Read the model definition and answer for the solid it produces. Units are mm, in the model's axes. A direction names the side the tool comes from. Coordinates: 2 decimals unless noted, no trailing zeros. Order: outer loops, then holes, each group sorted by start corner. A loop starts at its lowest first (then second) coordinate and runs counter-clockwise, first axis right, second up. Notation, with made-up numbers: (7.25, 0) -> (42.25, 0) arc R27 cw to (42.25, 23) -> close; hole circle Ø3 at (6.25, 19.25). An arc over 180 degrees is marked (long way). Answer as a JSON object with one key per item and string values. Group by question number.
1) Section D-D on x = 1 is taken. Determine the outline of the cut face in (y, z) (3 decimals), and give its area (3 significant figures).
2) A tool of negligible diameter and unlimited length cuts with its end or side. For faces 1 (the flat face through (1.5, 2.4, 9.2)), 2 (the flat face through (3, 2.875, 10)), 3 (the flat face through (5, 2.4, 9.2)), 4 (the flat face through (3, -2.375, 10)), from which of +Z, -Z, +X, -X, +Y, -Y can it reach the whole face along a straight path? Write none if from no direction.
3) Section A-A on z = -3.95 is taken. Determine the outline of the cut face in (x, y) (3 decimals).
4) Consider L1, parallel to Z at x = 5.25, y = 0; L2, parallel to Y at x = 2, z = -3.95 (3 decimals); L3, parallel to Y at x = 4.5, z = 6.75 (3 decimals). Determine where each line is inside the solid, lowest interval first.
5) Section B-B on x = 2.75 is taken. Determine the outline of the cut face in (y, z) (3 decimals), and give its area (3 significant figures).
6) Section C-C on y = 0 is taken. Determine the outline of the cut face in (x, z).
7) Determine the mould class of faces 5 (the flat face through (3, 1.875, 10)), 6 (the cylindrical face through (4.715, 2.368, 12.649)), 7 (the flat face through (3, 0, -6.45)), 8 (the cylindrical face through (3.204, -0.217, -2.974)) for opening direction Z: released by +Z, released by -Z, zero draft, split by the parting line, or undercut.
8) Given pin 1 (3 mm diameter, centred on x = 3, z = 8.5, fed in from -Y) (3 decimals); pin 2 (1.8 mm diameter, centred on x = 3.5, z = 9.5, fed in from +Y) (3 decimals); pin 3 (1.1 mm diameter, centred on y = -2.5, z = 8.5, fed in from +X), each flat-ended and moving along its own axis, determine where each tip first touches the part or whether it passes through.
Autodesk Inventor part; units mm, degrees
ref_plane "YZ Plane" through (0, 0, 0) normal (1, 0, 0) x (0, 1, 0)
ref_plane "XZ Plane" through (0, 0, 0) normal (0, 1, 0) x (-1, 0, 0)
ref_plane "XY Plane" through (0, 0, 0) normal (0, 0, 1) x (1, 0, 0)
sketch "Sketch1" plane through (0, 0, 0) normal (1, 0, 0) x (0, 1, 0)
  line L0 (6.375, 6.45) -> (-6.375, 6.45)
  line L1 (-6.375, 6.45) -> (-6.375, -6.45)
  line L2 (-6.375, -6.45) -> (6.375, -6.45)
  line L3 (6.375, -6.45) -> (6.375, 6.45)
  line L4 (6.375, 6.45) -> (-6.375, -6.45) construction
  line L5 (-6.375, 6.45) -> (6.375, -6.45) construction
  circle A0 centre (0, -3.95) radius 1
  circle A1 centre (0, 3.95) radius 1
  line L6 (0, 6.45) -> (0, -6.45)
  point P0 (0, 0)
  dimension "d0" = 12.75
  dimension "d1" = 12.9
  dimension "d2" = 2
  dimension "d3" = 2.5
  dimension "d4" = 2
  dimension "d5" = 2.5
extrude "Extrusion1" add sketch "Sketch1" along normal blind 6.5 contours L3 L2 L6 A0 A1 L0 | L6 A1 A0 L2 L1 L0
sketch "Sketch2" plane through (0, -6.375, 6.45) normal (0, 0, 1) x (1, 0, 0)
  line L0 (1.5, 9.25) -> (5, 9.25)
  line L1 (5, 9.25) -> (5, 8.25)
  line L2 (5, 8.25) -> (1.5, 8.25)
  line L3 (1.5, 8.25) -> (1.5, 9.25)
  line L4 (1.5, 9.25) -> (5, 8.25) construction
  line L5 (5, 9.25) -> (1.5, 8.25) construction
  line L6 (1.5, 4) -> (5, 4)
  line L7 (5, 4) -> (5, 3)
  line L8 (5, 3) -> (1.5, 3)
  line L9 (1.5, 3) -> (1.5, 4)
  line L10 (1.5, 4) -> (5, 3) construction
  line L11 (5, 4) -> (1.5, 3) construction
  line L12 (0, 12.75) -> (6.5, 12.75)
  line L13 (3.25, 12.75) -> (3.25, 0)
  line L14 (0, 0) -> (6.5, 0)
  point P0 (0, 6.375)
  point P1 (3.25, 8.75)
  point P2 (3.25, 3.5)
  point P3 (3.25, 8.75)
  point P4 (3.25, 3.5)
  dimension "d8" = 3.5
  dimension "d9" = 1
  dimension "d12" = 3.5
  dimension "d13" = 3.5
extrude "Extrusion2" add sketch "Sketch2" along normal blind 6.5
fillet "Fillet1" radius 1 4 edges at (5, 2.375, 12.95) (1.5, 2.375, 12.95) (1.5, -2.875, 12.95) (5, -2.875, 12.95)
properties part number "Switch"
Worked answers:
{
 "1": {"outline": "(-6.375, -6.45) -> (6.375, -6.45) -> (6.375, 6.45) -> (-6.375, 6.45) -> close; hole circle Ø2 at (0, -3.95); hole circle Ø2 at (0, 3.95)", "area": "158 mm²"},
 "2": {"face 1": "+Z, -X, +Y, -Y", "face 2": "+Z, +X, -X, +Y", "face 3": "+Z, +X, +Y, -Y", "face 4": "+Z, +X, -X"},
 "3": {"outline": "(0, -6.375) -> (6.5, -6.375) -> (6.5, -1) -> (0, -1) -> close; (0, 1) -> (6.5, 1) -> (6.5, 6.375) -> (0, 6.375) -> close"},
 "4": {"L1": "z = -6.45 to -4.95, -2.95 to 2.95, 4.95 to 6.45", "L2": "y = -6.375 to -1, 1 to 6.375", "L3": "y = -3.375 to -2.375, 1.875 to 2.875"},
 "5": {"outline": "(-6.375, -6.45) -> (6.375, -6.45) -> (6.375, 6.45) -> (2.875, 6.45) -> (2.875, 12.95) -> (1.875, 12.95) -> (1.875, 6.45) -> (-2.375, 6.45) -> (-2.375, 12.95) -> (-3.375, 12.95) -> (-3.375, 6.45) -> (-6.375, 6.45) -> close; hole circle Ø2 at (0, -3.95); hole circle Ø2 at (0, 3.95)", "area": "171 mm²"},
 "6": {"outline": "(0, -6.45) -> (6.5, -6.45) -> (6.5, -4.95) -> (0, -4.95) -> close; (0, -2.95) -> (6.5, -2.95) -> (6.5, 2.95) -> (0, 2.95) -> close; (0, 4.95) -> (6.5, 4.95) -> (6.5, 6.45) -> (0, 6.45) -> close"},
 "7": {"face 5": "zero draft", "face 6": "released by +Z", "face 7": "released by -Z", "face 8": "undercut"},
 "8": {"pin 1": "stops at y = -3.375", "pin 2": "stops at y = 2.875", "pin 3": "stops at x = 5"}
}
